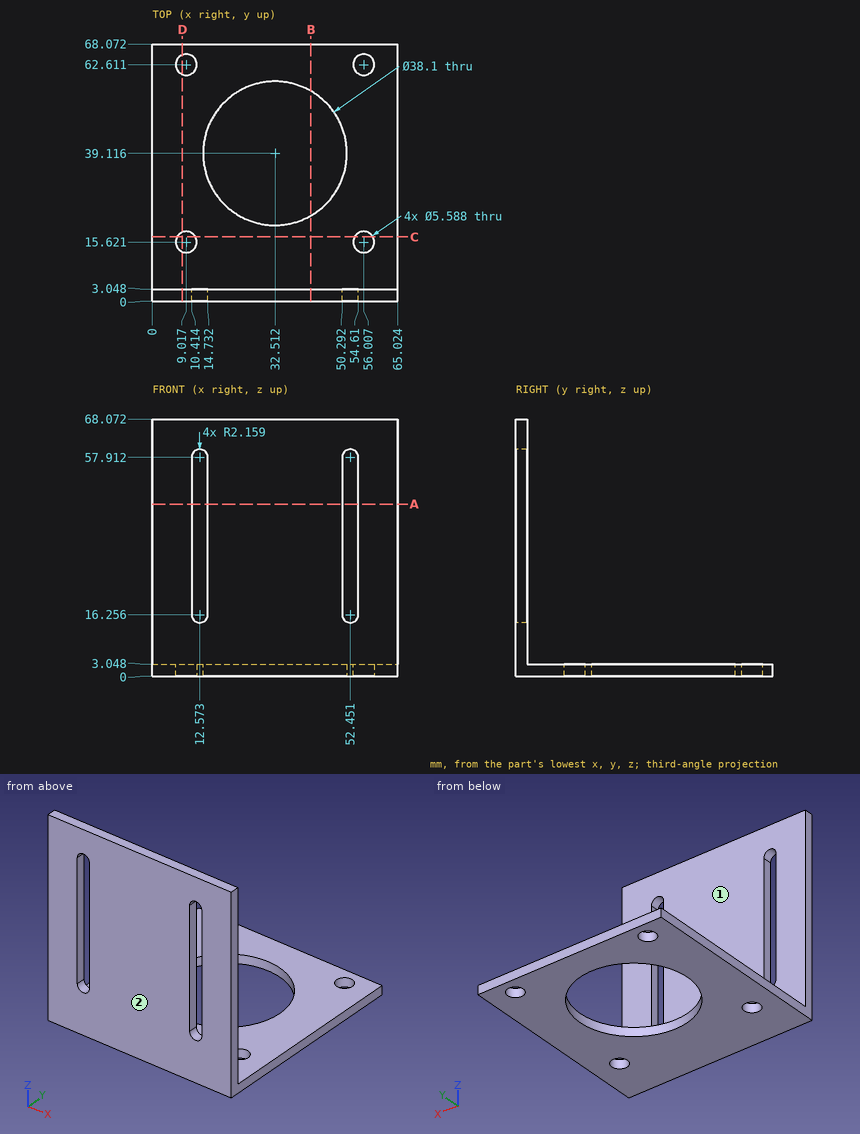
Can you work these out from the drawing? Everything is in mm from the part's minimum corner. A direction names the side the tool comes from. Coordinates: 2 decimals unless noted, no trailing zeros. Write each loop counter-clockwise with the first axis right and the second up, starting at its lowest first coordinate (ties: lowest second). Pieces come first, ordered by that corner, then holes. Notation, with made-up numbers: (73, 75) -> (109, 75) arc R18 ccw to (109, 108) -> close; hole circle Ø6 at (28, 16). An arc over 180 degrees is marked (long way). Return JSON: item names as keys, results as strings.
(1) Imagine slicing it at D-D, the plane x = 8. Please give me the cut outline in (y, z), then the cut area to 3 significant figures.
Numbers:
{"outline": "(0, 0) -> (13.02, 0) -> (13.02, 3.05) -> (3.05, 3.05) -> (3.05, 68.07) -> (0, 68.07) -> close; (18.22, 0) -> (60.01, 0) -> (60.01, 3.05) -> (18.22, 3.05) -> close; (65.21, 0) -> (68.07, 0) -> (68.07, 3.05) -> (65.21, 3.05) -> close", "area": "374 mm2"}
(2) Imagine slicing it at B-B, the plane x = 42. Please give me the cut outline in (y, z), then the cut area to 3 significant figures.
Numbers:
{"outline": "(0, 0) -> (22.6, 0) -> (22.6, 3.05) -> (3.05, 3.05) -> (3.05, 68.07) -> (0, 68.07) -> close; (55.64, 0) -> (68.07, 0) -> (68.07, 3.05) -> (55.64, 3.05) -> close", "area": "305 mm2"}
(3) Imagine slicing it at A-A, the plane z = 45.5. Please give me the cut outline in (x, y).
Numbers:
{"outline": "(0, 0) -> (10.41, 0) -> (10.41, 3.05) -> (0, 3.05) -> close; (14.73, 0) -> (50.29, 0) -> (50.29, 3.05) -> (14.73, 3.05) -> close; (54.61, 0) -> (65.02, 0) -> (65.02, 3.05) -> (54.61, 3.05) -> close"}
(4) I need wall thicknesses on L1, parallel to Y at x = 40, z = 37. Which ranges of the line are inside material? Lowest first, please.
Numbers:
{"L1": "y = 0 to 3.05"}
(5) Imagine slicing it at C-C, the plane y = 17. Please give me the cut outline in (x, z).
Numbers:
{"outline": "(0, 0) -> (6.59, 0) -> (6.59, 3.05) -> (0, 3.05) -> close; (11.45, 0) -> (53.58, 0) -> (53.58, 3.05) -> (11.45, 3.05) -> close; (58.44, 0) -> (65.02, 0) -> (65.02, 3.05) -> (58.44, 3.05) -> close"}
(6) Which directions (+Z, -Z, +X, -X, +Y, -Y) give clear straight access to the entire face, cutting with the end or side of a thin tool? Please do the marked faces 1 and 2.
Numbers:
{"face 1": "+Z, +X, -X, +Y", "face 2": "+Z, -Z, +X, -X, -Y"}
(7) I'm going to push flat-ended pins straight in: pin 1 (19.5 mm diameter, centred on x = 45, z = 49.5, fed in from +Y); pin 2 (3.5 mm diameter, centred on y = 2, z = 43.5, fed in from -X); pin 3 (8 mm diameter, centred on y = 14, z = 10, fed in from -X); pin 4 (19.5 mm diameter, centred on x = 31.5, y = 49, fed in from +Z). Where does each tip first touch, or does it pass through?
Numbers:
{"pin 1": "stops at y = 3.05", "pin 2": "stops at x = 0", "pin 3": "passes through", "pin 4": "stops at z = 3.05"}
